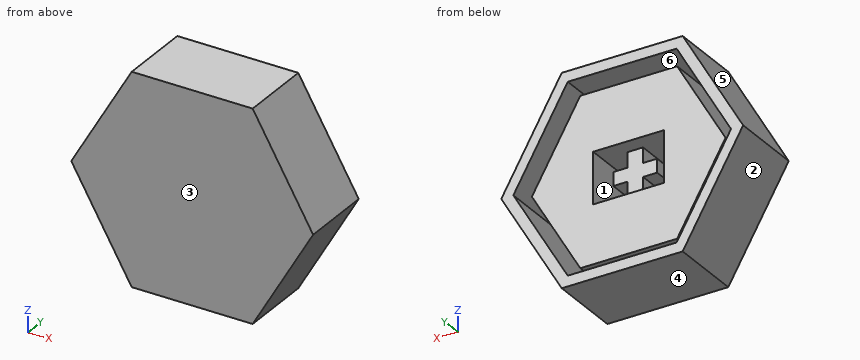
from build123d import *

# Parameters (mm, degrees)
BOSS_EXTRUDE1_DEPTH = 1
BOSS_EXTRUDE2_DEPTH = 7
SKETCH3_W           = 6.8
SKETCH3_H           = 4.9
BOSS_EXTRUDE3_DEPTH = 5
BOSS_EXTRUDE4_DEPTH = 4


with BuildPart() as part:
    # Sketch1 → Boss-Extrude1 (new body)
    with BuildSketch(Plane(origin=(0, 0, 0), x_dir=(1, 0, 0), z_dir=(0, 1, 0))):
        Polygon((10.421172359, 0), (5.210586179, 9.025), (-5.210586179, 9.025), (-10.421172359, 0), (-5.210586179, -9.025), (5.210586179, -9.025), align=None)
    extrude(amount=BOSS_EXTRUDE1_DEPTH)



with BuildPart() as body_2:
    # Sketch2 → Boss-Extrude2 (new body)
    with BuildSketch(Plane.XZ):
        Polygon((11.575872897, 0), (5.787936449, 10.025), (-5.787936449, 10.025), (-11.575872897, 0), (-5.787936449, -10.025), (5.787936449, -10.025), align=None)
        Polygon((10.421172359, 0), (5.210586179, 9.025), (-5.210586179, 9.025), (-10.421172359, 0), (-5.210586179, -9.025), (5.210586179, -9.025), align=None, mode=Mode.SUBTRACT)
    extrude(amount=-BOSS_EXTRUDE2_DEPTH)


with BuildPart() as part_1:
    add(part.part)

    add(body_2.part)  # Boss-Extrude3 merges body 2
    # Sketch3 → Boss-Extrude3 (add)
    with BuildSketch(Plane(origin=(0, 1, 0), x_dir=(1, 0, 0), z_dir=(0, 1, 0))):
        Polygon((4.63323591, -8.025), (9.26647182, 0), (4.63323591, 8.025), (-4.63323591, 8.025), (-9.26647182, 0), (-4.63323591, -8.025), align=None)
        Rectangle(SKETCH3_W, SKETCH3_H, mode=Mode.SUBTRACT)
    extrude(amount=BOSS_EXTRUDE3_DEPTH)

    # Sketch4 → Boss-Extrude4 (add)
    with BuildSketch(Plane(origin=(0, 1, 0), x_dir=(1, 0, 0), z_dir=(0, 1, 0))):
        Polygon((-0.75, 2.1), (0.75, 2.1), (0.75, 0.65), (2.1, 0.65), (2.1, -0.65), (0.75, -0.65), (0.75, -2.1), (-0.75, -2.1), (-0.75, -0.65), (-2.1, -0.65), (-2.1, 0.65), (-0.75, 0.65), align=None)
    extrude(amount=BOSS_EXTRUDE4_DEPTH)


solid = part_1.part
Check sheet for the modelled part. Datum: model origin and axes. Units: mm. Face numbers are marked on the shaded views. A direction names the side the tool comes from. Round coordinates to 2 decimals unless told otherwise and drop trailing zeros. Order: outer loops, then holes, each group sorted by start corner. A loop starts at its lowest first (then second) coordinate and runs counter-clockwise, first axis right, second up. Notation, with made-up numbers: M -13.75,31 L 23.25,31 A30 cw 23.25,60 Z; hole C -38.75,89.25 d10. An arc over 180 degrees is marked long. One line per item, written item: value. Start each with the question number.
1. Section check D-D on x = -3. Enter the section's corners in (y, z) (3 decimals).
2. Release check for a two-part mould opening along Z. For the marked faces 3, 4, 5 and 6 record: released by +Z, released by -Z, zero draft, split by the parting line, or undercut.
3. Section check B-B on x = 1.5. Enter the section's corners in (y, z) (3 decimals).
4. Scan lines: line 1 along Z through (x, y) = (-1.75, 4.5) (3 decimals); line 2 along Z through (x, y) = (3.5, 2.25) (3 decimals); line 3 along Z through (x, y) = (-0.25, 4.5) (3 decimals). Record each from-to range of solid material in increasing order.
5. Gauge pin test, flat ends, axial feed: P1, Ø2.5, axis at y = 2.5, z = -1, coming from the -X side; P2, Ø0.7, axis at y = 2.5, z = -1, coming from the -X side; P3, Ø3, axis at x = 2, z = 5.5, coming from the +Y side; P4, Ø2.5, axis at x = 1.5, z = -1, coming from the +Y side. Record the tip position at first contact, or that the pin passes through.
6. Access from +Z, -Z, +X, -X, +Y, -Y to the whole of each face (thin tool, end or side, straight path). Record for the marked faces 1 and 2.
7. Section check A-A on y = 4.25. Give the number of separate pieces and of enclosed holes in the cut face, and give its area (3 significant figures).
8. Section check C-C on z = 1.25. Enter the section's corners in (x, y), and give its area (3 significant figures).
Results found:
1. outline: M 0,-10.025 L 7,-10.025 L 7,-9.025 L 1,-9.025 L 1,-8.025 L 6,-8.025 L 6,-2.45 L 1,-2.45 L 1,2.45 L 6,2.45 L 6,8.025 L 1,8.025 L 1,9.025 L 7,9.025 L 7,10.025 L 0,10.025 Z
2. face 3: zero draft
2. face 4: released by -Z
2. face 5: released by +Z
2. face 6: undercut
3. outline: M 0,-10.025 L 7,-10.025 L 7,-9.025 L 1,-9.025 L 1,-8.025 L 6,-8.025 L 6,-2.45 L 1,-2.45 L 1,-0.65 L 5,-0.65 L 5,0.65 L 1,0.65 L 1,2.45 L 6,2.45 L 6,8.025 L 1,8.025 L 1,9.025 L 7,9.025 L 7,10.025 L 0,10.025 Z
4. line 1: -10.025 to -9.025, -8.025 to -2.45, -0.65 to 0.65, 2.45 to 8.025, 9.025 to 10.025
4. line 2: -10.025 to -9.025, -8.025 to 8.025, 9.025 to 10.025
4. line 3: -10.025 to -9.025, -8.025 to -2.45, -2.1 to 2.1, 2.45 to 8.025, 9.025 to 10.025
5. P1: x = -11.58
5. P2: x = -11.2
5. P3: y = 6
5. P4: y = 5
6. face 1: +Y
6. face 2: -Z, -X, +Y, -Y
7. separate pieces: 3
7. enclosed holes: 2
7. area: 266 mm^2
8. outline: M -10.85,0 L 10.85,0 L 10.85,7 L 9.7,7 L 9.7,1 L 8.54,1 L 8.54,6 L 3.4,6 L 3.4,1 L 0.75,1 L 0.75,5 L -0.75,5 L -0.75,1 L -3.4,1 L -3.4,6 L -8.54,6 L -8.54,1 L -9.7,1 L -9.7,7 L -10.85,7 Z
8. area: 93.0 mm^2
